Read the model definition and answer for the solid it produces. Units are mm, in the model's axes. Give positions to 0.01 mm unless a question says otherwise; leave off trailing zeros. Order: outer loops, then holes, each group sorted by start corner. A loop starts at its lowest first (then second) coordinate and runs counter-clockwise, first axis right, second up. Notation, with made-up numbers: (-23.5, 59) - (-8.5, 59) arc R11 ccw to (-8.5, 80) - close; hole circle Ø10 at (42, 50.25). An arc over 180 degrees is marked (long way). Write each question's results on one line, items separated by ' | '. Start each with the question number.
Q1. Find section B-B on z = 275. Give the vertices of the cut face in (x, y), and give its area (3 significant figures).
Q2. Find section A-A on y = 3. Give the vertices of the cut face in (x, z) (3 decimals).
Q3. Find the intervals of material crossed by line 1 along Z through (x, y) = (9.5, -19.5); line 2 along Y through (x, z) = (11.25, 304); line 3 along Y through (x, z) = (1.75, 307), in increasing order. Write a range as from..to.
Q4. Flat-ended cylindrical pins translate along their axes: P1, Ø6, axis at x = 3, y = -4.5, coming from the -Z side; P2, Ø4, axis at x = 4.5, y = 7, coming from the +Z side (3 decimals); P3, Ø1.5, axis at x = 13, y = -30.5, coming from the +Z side. Find the tip coordinate at first contact, or state that the pin passes through.
from build123d import *

# Parameters (mm, degrees)
EXTRUDE_1_DEPTH = 16
FILLET_1_R      = 3


with BuildPart() as part:
    # 草图1 → 凸台-拉伸1 (new body)
    with BuildSketch(Plane(origin=(0, 0, 0), x_dir=(0, 0, -1), z_dir=(1, 0, 0))):
        with BuildLine():
            Line((-375, 18), (-42.332020977, 18))
            ThreePointArc((-42.332020977, 18), (-38.366652187, -25.377155081), (0, -46))
            Line((0, -46), (-255, -46))
            Line((-255, -46), (-375, 18))
        make_face()
    extrude(amount=EXTRUDE_1_DEPTH)

    # 圆角1
    fillet_1_edges = [part.edges().sort_by_distance(p)[0] for p in [
        (8, 18, 375),
        (8, -46, 0),
    ]]
    fillet(fillet_1_edges, radius=FILLET_1_R)


solid = part.part
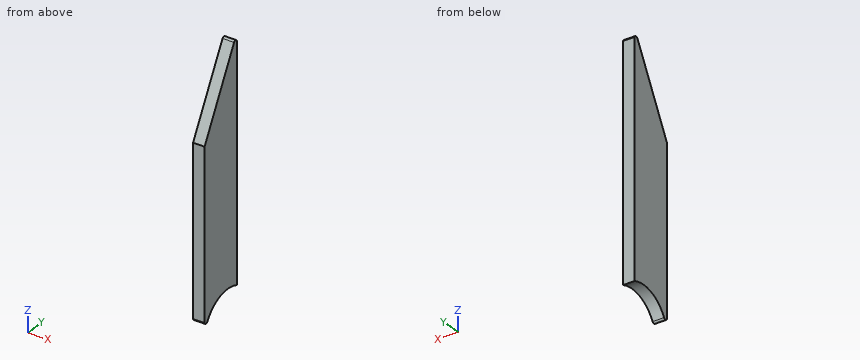
Working result:
1) outline: (0, -35.33) - (16, -35.33) - (16, 18) - (0, 18) - close | area: 853 mm²
2) outline: (0, 45.902) - (16, 45.902) - (16, 346.875) - (0, 346.875) - close
3) line 1: 41.66..304.69 | line 2: -19.87..18 | line 3: -18.27..18
4) P1: z = 45.38 | P2: z = 358.125 | P3: z = 285.47
